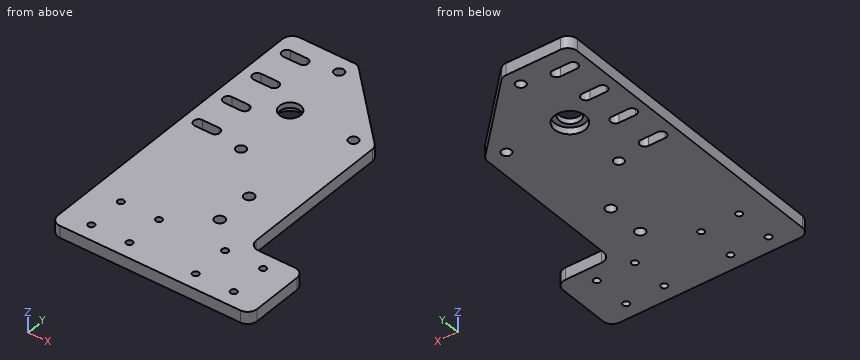
from build123d import *

# Parameters (mm, degrees)
CROQUIS1_R          = 1.7
CROQUIS1_R_2        = 2.65
CROQUIS1_R_3        = 5.5
CROQUIS1_R_4        = 2.55
EXTRUDE_1_DEPTH     = 6.35
EXTRUDE_START       = -6.35
CROQUIS2_R          = 8.025
EXTRUDE_CUT_1_DEPTH = 3.5


with BuildPart() as part:
    # Croquis1 → Extrude 1 (new body)
    with BuildSketch(Plane.XY):
        with BuildLine():
            Line((-65, -34), (-65, 86.95))
            ThreePointArc((-65, 86.95), (-63.535533906, 90.485533906), (-60, 91.95))
            Line((-60, 91.95), (-31.351067812, 91.95))
            ThreePointArc((-31.351067812, 91.95), (-29.43765065, 91.569397663), (-27.815533906, 90.485533906))
            Line((-27.815533906, 90.485533906), (9.255533906, 53.414466094))
            ThreePointArc((9.255533906, 53.414466094), (10.339397663, 51.79234935), (10.72, 49.878932188))
            Line((10.72, 49.878932188), (10.72, -29))
            ThreePointArc((10.72, -29), (12.184466094, -32.535533906), (15.72, -34))
            Line((15.72, -34), (34.8, -34))
            ThreePointArc((34.8, -34), (38.335533906, -35.464466094), (39.8, -39))
            Line((39.8, -39), (39.8, -66))
            ThreePointArc((39.8, -66), (38.335533906, -69.535533906), (34.8, -71))
            Line((34.8, -71), (-60, -71))
            ThreePointArc((-60, -71), (-63.535533906, -69.535533906), (-65, -66))
            Line((-65, -66), (-65, -34))
        make_face()
        with Locations((-50, -42.5)):
            Circle(CROQUIS1_R, mode=Mode.SUBTRACT)
        with Locations((-30, -42.5)):
            Circle(CROQUIS1_R, mode=Mode.SUBTRACT)
        with Locations((-30, -62.5)):
            Circle(CROQUIS1_R, mode=Mode.SUBTRACT)
        with Locations((-50, -62.5)):
            Circle(CROQUIS1_R, mode=Mode.SUBTRACT)
        with Locations((4.8, -62.5)):
            Circle(CROQUIS1_R, mode=Mode.SUBTRACT)
        with Locations((4.8, -42.5)):
            Circle(CROQUIS1_R, mode=Mode.SUBTRACT)
        with Locations((24.8, -42.5)):
            Circle(CROQUIS1_R, mode=Mode.SUBTRACT)
        with Locations((24.8, -62.5)):
            Circle(CROQUIS1_R, mode=Mode.SUBTRACT)
        with Locations((-10, -7)):
            Circle(CROQUIS1_R_2, mode=Mode.SUBTRACT)
        with Locations((-10, -27)):
            Circle(CROQUIS1_R_2, mode=Mode.SUBTRACT)
        with Locations((-32.55, 50)):
            Circle(CROQUIS1_R_3, mode=Mode.SUBTRACT)
        with Locations((-32.55, 16.666986335)):
            Circle(CROQUIS1_R_4, mode=Mode.SUBTRACT)
        with Locations((-32.55, 83.333013665)):
            Circle(CROQUIS1_R_4, mode=Mode.SUBTRACT)
        with Locations((0.783013665, 50)):
            Circle(CROQUIS1_R_4, mode=Mode.SUBTRACT)
        with BuildLine():
            Line((-57.45, 22.55), (-48.75, 22.55))
            ThreePointArc((-48.75, 22.55), (-46.2, 20), (-48.75, 17.45))
            Line((-48.75, 17.45), (-57.45, 17.45))
            ThreePointArc((-57.45, 17.45), (-60, 20), (-57.45, 22.55))
        make_face(mode=Mode.SUBTRACT)
        with BuildLine():
            Line((-57.45, 82.55), (-48.75, 82.55))
            ThreePointArc((-48.75, 82.55), (-46.2, 80), (-48.75, 77.45))
            Line((-48.75, 77.45), (-57.45, 77.45))
            ThreePointArc((-57.45, 77.45), (-60, 80), (-57.45, 82.55))
        make_face(mode=Mode.SUBTRACT)
        with BuildLine():
            Line((-57.45, 62.55), (-48.75, 62.55))
            ThreePointArc((-48.75, 62.55), (-46.2, 60), (-48.75, 57.45))
            Line((-48.75, 57.45), (-57.45, 57.45))
            ThreePointArc((-57.45, 57.45), (-60, 60), (-57.45, 62.55))
        make_face(mode=Mode.SUBTRACT)
        with BuildLine():
            Line((-57.45, 42.55), (-48.75, 42.55))
            ThreePointArc((-48.75, 42.55), (-46.2, 40), (-48.75, 37.45))
            Line((-48.75, 37.45), (-57.45, 37.45))
            ThreePointArc((-57.45, 37.45), (-60, 40), (-57.45, 42.55))
        make_face(mode=Mode.SUBTRACT)
    extrude(amount=EXTRUDE_1_DEPTH)

    # Croquis2 → Extrude Cut 1 (cut)
    with BuildSketch(Plane.XY.offset(6.35).offset(EXTRUDE_START)):
        with Locations(Location((-32.55, 50, 0), (0, 0, 180))):
            Circle(CROQUIS2_R)
    extrude(amount=EXTRUDE_CUT_1_DEPTH, mode=Mode.SUBTRACT)


solid = part.part
Check sheet for the modelled part. Datum: model origin and axes. Units: mm. Round coordinates to 2 decimals unless told otherwise and drop trailing zeros. Write each loop counter-clockwise with the first axis right and the second up, starting at its lowest first coordinate (ties: lowest second). Pieces come first, ordered by that corner, then holes. Notation, with made-up numbers: (-36.5, -8) -> (-10.5, -8) arc R28 ccw to (-10.5, 30) -> close; hole circle Ø2 at (75.5, 63.25). An arc over 180 degrees is marked (long way). Answer as CSV lines item,"result". Start each with the question number.
1) Section check C-C on x = -10.5. Enter the section's corners in (y, z), and give its area (3 significant figures).
2) Section check B-B on y = -42.5. Enter the section's corners in (x, z), and give its area (3 significant figures).
3) Material ranges on line 1 (Y direction, x = 24.8, z = 3.75); line 2 (Y direction, x = 4.8, z = 3.75); line 3 (Y direction, x = -32.55, z = 2.75) (3 decimals), recorded low to high. Write a range as from..to.
4) Section check D-D on x = -21. Enter the section's corners in (y, z).
5) Go/stop test with flat-tipped pins: P1, Ø4.5, axis at x = 24.8, y = -62.5, coming from the -Z side; P2, Ø3, axis at x = -25, z = 3, coming from the +Y side. Record where each tip stops, or that it passes through.
6) Section check A-A on y = 60. Enter the section's corners in (x, z).
Found:
1,outline,"(-71, 0) -> (-29.6, 0) -> (-29.6, 6.35) -> (-71, 6.35) -> close; (-24.4, 0) -> (-9.6, 0) -> (-9.6, 6.35) -> (-24.4, 6.35) -> close; (-4.4, 0) -> (73.17, 0) -> (73.17, 6.35) -> (-4.4, 6.35) -> close"
1,area,"849 mm^2"
2,outline,"(-65, 0) -> (-51.7, 0) -> (-51.7, 6.35) -> (-65, 6.35) -> close; (-48.3, 0) -> (-31.7, 0) -> (-31.7, 6.35) -> (-48.3, 6.35) -> close; (-28.3, 0) -> (3.1, 0) -> (3.1, 6.35) -> (-28.3, 6.35) -> close; (6.5, 0) -> (23.1, 0) -> (23.1, 6.35) -> (6.5, 6.35) -> close; (26.5, 0) -> (39.8, 0) -> (39.8, 6.35) -> (26.5, 6.35) -> close"
2,area,"579 mm^2"
3,line 1,"y = -71..-64.2, -60.8..-44.2, -40.8..-34"
3,line 2,"y = -71..-64.2, -60.8..-44.2, -40.8..57.87"
3,line 3,"y = -71..14.117, 19.217..41.975, 58.025..80.783, 85.883..91.95"
4,outline,"(-71, 0) -> (83.67, 0) -> (83.67, 6.35) -> (-71, 6.35) -> close"
5,P1,"stops at z = 0"
5,P2,"stops at y = 89.17"
6,outline,"(-65, 0) -> (-60, 0) -> (-60, 6.35) -> (-65, 6.35) -> close; (-46.2, 0) -> (2.67, 0) -> (2.67, 6.35) -> (-46.2, 6.35) -> close"
